For this review, take the finished solid that the model builds, in its own axes (mm). Face numbers are marked on the shaded views. A direction names the side the tool comes from. Round coordinates to 2 decimals unless told otherwise and drop trailing zeros. Write each loop counter-clockwise with the first axis right and the second up, starting at its lowest first coordinate (ties: lowest second). Pieces come first, ordered by that corner, then holes. Notation, with made-up numbers: M 55.25,-36.75 L 91.25,-36.75 A30 ccw 91.25,-1.75 Z; hole C 73,-17 d6. An arc over 180 degrees is marked long. One line per question, with ' | ' between items.
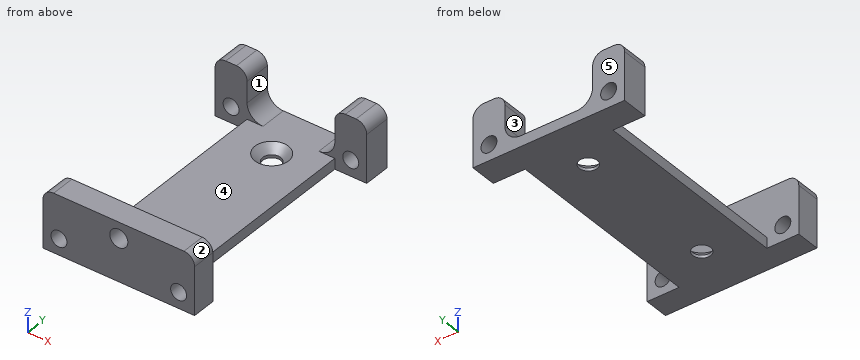
Autodesk Inventor part; units mm, degrees
ref_plane "Work Plane1" through (-9.075, -7.1151, 3.005) normal (0, 1, 0) x (0, 0, 1)
ref_plane "YZ Plane" through (0, 0, 0) normal (1, 0, 0) x (0, 1, 0)
ref_plane "XZ Plane" through (0, 0, 0) normal (0, 1, 0) x (-1, 0, 0)
sketch "Sketch1" plane through (0, 0, 0) normal (0, 0, 1) x (1, 0, 0)
  line L0 (-14.25, -23.75) -> (14.25, -23.75)
  line L1 (14.25, -23.75) -> (14.25, 23.75)
  line L2 (14.25, 23.75) -> (-14.25, 23.75)
  line L3 (-14.25, 23.75) -> (-14.25, -23.75)
  line L4 (-14.25, -23.75) -> (14.25, 23.75) construction
  line L5 (14.25, -23.75) -> (-14.25, 23.75) construction
  line L6 (-14.25, 18.75) -> (14.25, 18.75)
  line L7 (-14.25, -19.25) -> (14.25, -19.25)
  line L8 (-8.25, 18.75) -> (-8.25, -19.25)
  line L9 (8.25, 18.75) -> (8.25, -19.25)
  point P0 (0, 0)
  dimension "d0" = 28.5
  dimension "d1" = 47.5
  dimension "d36" = 4.5
  dimension "d37" = 5
  dimension "d38" = 6
  dimension "d39" = 6
extrude "Extrusion1" add sketch "Sketch1" along normal blind 2 contours L3 L7 L1 L0 | L3 L2 L1 L6 | L8 L6 L9 L7
sketch "Sketch2" plane through (0, 0, 2) normal (0, 0, 1) x (1, 0, 0)
  line L0 (-14.25, 23.75) -> (-14.25, -23.75)
  line L1 (14.25, -23.75) -> (14.25, 23.75)
  line L2 (-14.25, -23.75) -> (14.25, -23.75)
  line L3 (14.25, -23.75) -> (14.25, -19.25)
  line L4 (14.25, -19.25) -> (-14.25, -19.25)
  line L5 (-14.25, -19.25) -> (-14.25, -23.75)
  line L6 (-14.25, 23.75) -> (14.25, 23.75)
  line L7 (14.25, 23.75) -> (14.25, 18.75)
  line L8 (14.25, 18.75) -> (-14.25, 18.75)
  line L9 (-14.25, 18.75) -> (-14.25, 23.75)
  point P0 (0, 0)
  point P1 (14.25, 23.75)
  dimension "d4" = 4.5
  dimension "d19" = 5
extrude "Extrusion2" add sketch "Sketch2" along normal blind 9 contours L6 L1 L8 L0 | L4 L1 L2 L0
sketch "Sketch3" plane through (-14.25, -23.75, 0) normal (0, -1, 0) x (1, 0, 0)
  line L0 (0, 11) -> (28.5, 11) construction
  line L1 (14.25, 11) -> (14.25, 0) construction
  line L2 (3, 3) -> (25.5, 3) construction
  line L3 (0, 0) -> (28.5, 0) construction
  point P0 (14.25, 3)
  dimension "d7" = 22.5
  dimension "d8" = 3
hole "Hole1" at (-11.25, -23.75, 3) at (11.25, -23.75, 3) direction (0, 1, 0) diameter 3 depth 46.5 tip angle 118
sketch "Sketch4" plane through (-14.25, -23.75, 0) normal (0, -1, 0) x (1, 0, 0)
  circle A0 centre (3, 3) radius 1.5 construction
  circle A1 centre (25.5, 3) radius 1.5 construction
  line L0 (3, 3) -> (25.5, 3) construction
  circle A2 centre (14.25, 8) radius 1.7
  line L1 (14.25, 8) -> (14.25, 3) construction
  point P0 (14.25, 0)
  dimension "d40" = 5
  dimension "d41" = 3.4
extrude "Extrusion3" cut sketch "Sketch4" against normal up to surface (4.5 mm away)
sketch "Sketch6" plane through (-14.25, 23.75, 0) normal (0, 1, 0) x (1, 0, 0)
  line L0 (22.5, -11) -> (6, -11)
  line L1 (6, -11) -> (6, -2)
  line L2 (6, -2) -> (22.5, -2)
  line L3 (22.5, -2) -> (22.5, -11)
  line L4 (22.5, -11) -> (6, -2) construction
  line L5 (6, -11) -> (22.5, -2) construction
  line L6 (14.25, 0) -> (14.25, -11) construction
  line L7 (28.5, -11) -> (0, -11) construction
  line L8 (22.5, -2) -> (6, -2) construction
  circle A0 centre (25.5, -3) radius 1.5
  circle A1 centre (3, -3) radius 1.5
  point P0 (14.25, -6.5)
  point P1 (14.25, -6.5)
extrude "Extrusion5" cut sketch "Sketch6" against normal up to surface (5 mm away)
fillet "Fillet1" radius 2 6 edges at (-14.25, 21.25, 11) (14.25, 21.25, 11) (-14.25, -21.5, 11) (14.25, -21.5, 11) (-8.25, 21.25, 11) (8.25, 21.25, 11)
fillet "Fillet2" radius 3 2 edges at (-8.25, 21.25, 2) (8.25, 21.25, 2)
ref_plane "Work Plane1" through (-9.075, -7.1151, 3.005) normal (0, 1, 0) x (0, 0, 1)
sketch "Sketch10" plane through (0, 0, 2) normal (0, 0, 1) x (1, 0, 0)
  line L0 (0, 14) -> (0, -14) construction
  point P0 (0, 0)
  point P1 (0, 0)
  dimension "d46" = 28
hole "Hole2" at (0, 14, 2) at (0, -14, 2) direction (0, 0, -1) diameter 3.4 depth 46.5 tip angle 118 countersink diameter 6.3 countersink angle 90
equation "\"d1\" = 1.66667 * d0"
equation "\"d39\" = d38"
properties part number "Tension_Bock"
Item 1: Insertion check: pin 1 Ø4 at (x, y) = (0, -14) entering from +Z; pin 2 Ø2.5 at (x, z) = (11.25, 3) entering from +Y; pin 3 Ø1 at (y, z) = (7.5, 1.5) entering from +X; pin 4 Ø0.6 at (y, z) = (0, 1.5) entering from -X. Each pin has a flat end and moves straight along its axis. Give the tip position at first contact, or say it passes through.
Results:
pin 1: z = 0.85 | pin 2: through | pin 3: x = 8.25 | pin 4: x = -8.25
Item 2: Machinability: for the marked faces 1 and 2, which of the approach directions +Z, -Z, +X, -X, +Y, -Y give a long, thin tool a straight path to every point of the face, cutting with its end or side? Answer none if there is none.
Results:
face 1: +Z, +Y | face 2: +Z, +X, +Y, -Y
Item 3: Take a section at B-B (y = -14). Write out the cut boundary in (x, z), then the cut area to 3 significant figures.
Results:
outline: M -8.25,0 L -1.7,0 L -1.7,0.55 L -3.15,2 L -8.25,2 Z; M 1.7,0 L 8.25,0 L 8.25,2 L 3.15,2 L 1.7,0.55 Z | area: 24.1 mm2
Item 4: Take a section at C-C (x = -7.75). Write out the cut boundary in (y, z).
Results:
outline: M -23.75,0 L 23.75,0 L 23.75,3.34 L 18.75,3.34 L 18.75,2 L -19.25,2 L -19.25,11 L -23.75,11 Z
Item 5: To check wall thickness, follow line 1 along X through (y, z) = (-20.95, 3); line 2 along Z through (x, y) = (-11.25, -20.55); line 3 along Y through (x, z) = (-9.5, 5). State the ranges of each line that lie inside material, in increasing order. Write a range as from..to.
Results:
line 1: -14.25..-12.75, -9.75..9.75, 12.75..14.25 | line 2: 0..1.5, 4.5..11 | line 3: -23.75..-19.25, 18.75..23.75
Item 6: Take a section at D-D (z = 3.75). Write out the cut boundary in (x, y), then the cut area to 3 significant figures.
Results:
outline: M -14.25,-23.75 L -12.55,-23.75 L -12.55,-19.25 L -14.25,-19.25 Z; M -14.25,18.75 L -12.55,18.75 L -12.55,23.75 L -14.25,23.75 Z; M -9.95,-23.75 L 9.95,-23.75 L 9.95,-19.25 L -9.95,-19.25 Z; M -9.95,18.75 L -7.98,18.75 L -7.98,23.75 L -9.95,23.75 Z; M 7.98,18.75 L 9.95,18.75 L 9.95,23.75 L 7.98,23.75 Z; M 12.55,-23.75 L 14.25,-23.75 L 14.25,-19.25 L 12.55,-19.25 Z; M 12.55,18.75 L 14.25,18.75 L 14.25,23.75 L 12.55,23.75 Z | area: 142 mm2
Item 7: Take a section at A-A (z = 8). Write out the cut boundary in (x, y), then the cut area to 3 significant figures.
Results:
outline: M -14.25,-23.75 L -1.7,-23.75 L -1.7,-19.25 L -14.25,-19.25 Z; M -14.25,18.75 L -8.25,18.75 L -8.25,23.75 L -14.25,23.75 Z; M 1.7,-23.75 L 14.25,-23.75 L 14.25,-19.25 L 1.7,-19.25 Z; M 8.25,18.75 L 14.25,18.75 L 14.25,23.75 L 8.25,23.75 Z | area: 173 mm2
Item 8: Mouldability with a two-part tool opening along Y and no side actions: class the marked faces 3, 4 and 5 as +Y half, -Y half, draft (parallel to the pull), parting line (faces both ways), or undercut.
Results:
face 3: draft | face 4: undercut | face 5: +Y half
